Autodesk Inventor part; units mm, degrees
ref_plane "YZ Plane" through (0, 0, 0) normal (1, 0, 0) x (0, 1, 0)
ref_plane "XZ Plane" through (0, 0, 0) normal (0, 1, 0) x (-1, 0, 0)
ref_plane "XY Plane" through (0, 0, 0) normal (0, 0, 1) x (1, 0, 0)
sketch "Boceto1" plane through (0, 0, 0) normal (0, 0, 1) x (1, 0, 0)
  circle A0 centre (0, 0) radius 1.65
  line L0 (-15.5, -10) -> (35.5, -10) construction
  line L1 (5, -10) -> (-5, -10)
  line L2 (-5, -10) -> (-5, 5)
  line L3 (-5, 5) -> (5, 5)
  line L4 (5, 5) -> (5, -10)
  line L5 (-15, -10) -> (15, -10)
  line L6 (15, -10) -> (15, -6)
  line L7 (15, -6) -> (-15, -6)
  line L8 (-15, -6) -> (-15, -10)
  point P0 (-5, -6)
  point P1 (5, -6)
  dimension "d0" = 3.3
  dimension "d1" = 5
  dimension "d2" = 5
  dimension "d3" = 5
  dimension "d4" = 10
  dimension "d5" = 10
  dimension "d6" = 4
extrude "Extrusión1" add sketch "Boceto1" along normal blind 1 and the other way blind 7 contours A0 | L1 L2 L7 L4 | L4 L7 L6 L5 | L5 L8 L7 L2 | L7 L2 L3 L4
sketch "Boceto2" plane through (-15, -6, -7) normal (0, 1, 0) x (-1, 0, 0)
  line L0 (-30, 0) -> (-20, 0) construction
  line L1 (-30, 0) -> (-30, 8) construction
  line L2 (0, 8) -> (-10, 8) construction
  line L3 (0, 0) -> (0, 8) construction
  line L4 (-20, 8) -> (-30, 8)
  point P0 (-15, 7)
  point P1 (-3, 3.5)
  point P2 (-27, 3.5)
  dimension "d35" = 3.5
  dimension "d36" = 3
  dimension "d37" = 3.5
  dimension "d38" = 3
hole "Agujero1" at (-12, -6, -3.5) at (12, -6, -3.5) direction (0, -1, 0) diameter 3.4 end through all
fillet "Empalme1" radius 5 2 edges at (-5, 5, -3) (5, 5, -3)
fillet "Empalme2" radius 3 2 edges at (-5, -6, -3) (5, -6, -3)
fillet "Empalme3" radius 1 4 edges at (-15, -8, -7) (-15, -8, 1) (15, -8, -7) (15, -8, 1)
sketch "Boceto6" plane through (0, 0, -7) normal (0, 0, -1) x (-1, 0, 0)
  point P0 (0, 0)
hole "Agujero3" at (0, 0, -7) direction (0, 0, 1) diameter 3.3 depth 7
properties part number "SoporteEjes"
Part model, mm, in its own coordinate system. A direction names the side the tool comes from. Round coordinates to 2 decimals unless told otherwise and drop trailing zeros. Write each loop counter-clockwise with the first axis right and the second up, starting at its lowest first coordinate (ties: lowest second). Pieces come first, ordered by that corner, then holes.
Item 1: Two-plate mould, pull along Z, no slides. Class faces 4 (the cylindrical face through (12.65, -8.03, -1.93)), 5 (the flat face through (0, 0, 0)), 6 (the cylindrical face through (-5.9, -5.14, -2.94)): +Z half, -Z half, draft (parallel to the pull), parting line (faces both ways), or undercut.
Results:
face 4: undercut
face 5: -Z half
face 6: draft
Item 2: Which spindle directions (+Z, -Z, +X, -X, +Y, -Y) get a long thin tool onto all of the face, cutting with end or side? Do faces 1 (the flat face through (-5, -2, -3)), 2 (the flat face through (5, -1, -3)), 3 (the cylindrical face through (-1.115, -1.216, -3.451)). Say none if no direction does.
Results:
face 1: +Z, -Z, -X, +Y
face 2: +Z, -Z, +X, +Y
face 3: -Z
Item 3: Cut at D-D, the plane x = 13. Give the cut face in (y, z), plus the area to 3 significant figures.
Results:
outline: (-10, -7) - (-6, -7) - (-6, -4.87) - (-10, -4.87) - close; (-10, -2.13) - (-6, -2.13) - (-6, 1) - (-10, 1) - close
area: 21.0 mm2
Item 4: Drop flat-ended pins along their axis: pin 1 Ø3 at (x, y) = (0, 0) entering from -Z; pin 2 Ø4 at (y, z) = (-3, -1.5) entering from +X; pin 3 Ø3.5 at (y, z) = (-2, -2) entering from -X; pin 4 Ø4.5 at (x, z) = (12, -3.5) entering from -Y. Give the stop position or say it passes through.
Results:
pin 1: stops at z = 0
pin 2: stops at x = 5.76
pin 3: stops at x = -5.1
pin 4: stops at y = -10
Item 5: Cut at B-B, the plane y = -7.25. Give the cut face in (x, z).
Results:
outline: (-15, -6) arc R1 ccw to (-14, -7) - (14, -7) arc R1 ccw to (15, -6) - (15, 0) arc R1 ccw to (14, 1) - (-14, 1) arc R1 ccw to (-15, 0) - close; hole circle Ø3.4 at (-12, -3.5); hole circle Ø3.4 at (12, -3.5)
Item 6: Cut at A-A, the plane z = -3.5. Count the separate pieces of the cut face and the enclosed holes in it, plus the area to 3 significant figures.
Results:
separate pieces: 3
enclosed holes: 1
area: 187 mm2
Item 7: Cut at C-C, the plane x = -12. Give the cut face in (y, z), plus the area to 3 significant figures.
Results:
outline: (-10, -7) - (-6, -7) - (-6, -5.2) - (-10, -5.2) - close; (-10, -1.8) - (-6, -1.8) - (-6, 1) - (-10, 1) - close
area: 18.4 mm2
Item 8: Probe L1, parallel to Z at x = -12, y = -8.3; L2, parallel to Y at x = -9.25, z = 0.75; L3, parallel to Y at x = -0.5, z = -1.75. List the from-to ranges inside material, lowest first.
Results:
L1: z = -7 to -5.2, -1.8 to 1
L2: y = -10 to -6
L3: y = -10 to -1.57, 1.57 to 4.97
